Here's how the part is built. I have some questions about the finished solid (model axes, mm). A direction names the side the tool comes from. Round coordinates to 2 decimals unless told otherwise and drop trailing zeros. Loops run counter-clockwise (first coordinate to the right, second up) from the corner with the lowest first, then second, coordinate; pieces in that order, holes last. Notation, with made-up numbers: (83, 65.5) -> (115, 65.5) arc R21 cw to (115, 104.5) -> close; hole circle Ø6 at (41, 47.5). An arc over 180 degrees is marked (long way). One line per item, written item: value. Start each with the question number.
```python
from build123d import *

# Parameters (mm, degrees)
SKETCH1_W            = 40
SKETCH1_H            = 40
BOSS_EXTRUDE1_DEPTH  = 687
SKETCH1_4_W          = 40
SKETCH1_4_H          = 40
BOSS_EXTRUDE2_DEPTH  = 687
SKETCH1_5_W          = 40
SKETCH1_5_H          = 40
BOSS_EXTRUDE3_DEPTH  = 687
SKETCH1_6_W          = 40
SKETCH1_6_H          = 40
BOSS_EXTRUDE4_DEPTH  = 687
SKETCH1_7_W          = 820
SKETCH1_7_H          = 40
BOSS_EXTRUDE5_DEPTH  = 40
SKETCH1_8_W          = 40
SKETCH1_8_H          = 520
BOSS_EXTRUDE6_DEPTH  = 40
SKETCH1_9_W          = 820
SKETCH1_9_H          = 40
BOSS_EXTRUDE7_DEPTH  = 40
SKETCH1_10_W         = 40
SKETCH1_10_H         = 520
BOSS_EXTRUDE8_DEPTH  = 40
BOSS_EXTRUDE9_DEPTH  = 40
BOSS_EXTRUDE10_DEPTH = 40
BOSS_EXTRUDE11_DEPTH = 40
BOSS_EXTRUDE12_DEPTH = 40
SKETCH6_W            = 40
SKETCH6_H            = 40
BOSS_EXTRUDE13_DEPTH = 820
SKETCH7_W            = 40
SKETCH7_H            = 40
BOSS_EXTRUDE14_DEPTH = 520
SKETCH8_W            = 40
SKETCH8_H            = 40
BOSS_EXTRUDE15_DEPTH = 520
SKETCH9_R            = 12.5
BOSS_EXTRUDE16_DEPTH = 9


with BuildPart() as part:
    # Sketch1 → Boss-Extrude1 (new body)
    with BuildSketch(Plane.XY):
        with Locations((20, 580)):
            Rectangle(SKETCH1_W, SKETCH1_H)
    extrude(amount=BOSS_EXTRUDE1_DEPTH)



with BuildPart() as body_2:
    # Sketch1_4 → Boss-Extrude2 (new body)
    with BuildSketch(Plane.XY):
        with Locations((880, 580)):
            Rectangle(SKETCH1_4_W, SKETCH1_4_H)
    extrude(amount=BOSS_EXTRUDE2_DEPTH)


with BuildPart() as body_3:
    # Sketch1_5 → Boss-Extrude3 (new body)
    with BuildSketch(Plane.XY):
        with Locations((20, 20)):
            Rectangle(SKETCH1_5_W, SKETCH1_5_H)
    extrude(amount=BOSS_EXTRUDE3_DEPTH)


with BuildPart() as body_4:
    # Sketch1_6 → Boss-Extrude4 (new body)
    with BuildSketch(Plane.XY):
        with Locations((880, 20)):
            Rectangle(SKETCH1_6_W, SKETCH1_6_H)
    extrude(amount=BOSS_EXTRUDE4_DEPTH)


with BuildPart() as part_1:
    add(part.part)

    add(body_2.part)  # Boss-Extrude5 merges body 2
    # Sketch1_7 → Boss-Extrude5 (add)
    with BuildSketch(Plane.XY):
        with Locations((450, 580)):
            Rectangle(SKETCH1_7_W, SKETCH1_7_H)
    extrude(amount=BOSS_EXTRUDE5_DEPTH)


    add(body_3.part)  # Boss-Extrude6 merges body 3
    # Sketch1_8 → Boss-Extrude6 (add)
    with BuildSketch(Plane.XY):
        with Locations((20, 300)):
            Rectangle(SKETCH1_8_W, SKETCH1_8_H)
    extrude(amount=BOSS_EXTRUDE6_DEPTH)


    add(body_4.part)  # Boss-Extrude7 merges body 4
    # Sketch1_9 → Boss-Extrude7 (add)
    with BuildSketch(Plane.XY):
        with Locations((450, 20)):
            Rectangle(SKETCH1_9_W, SKETCH1_9_H)
    extrude(amount=BOSS_EXTRUDE7_DEPTH)

    # Sketch1_10 → Boss-Extrude8 (add)
    with BuildSketch(Plane.XY):
        with Locations((880, 300)):
            Rectangle(SKETCH1_10_W, SKETCH1_10_H)
    extrude(amount=BOSS_EXTRUDE8_DEPTH)

    # Sketch2 → Boss-Extrude9 (add)
    with BuildSketch(Plane(origin=(0, 600, 0), x_dir=(1, 0, 0), z_dir=(0, 1, 0))):
        Polygon((40, -140), (140, -40), (40, -40), align=None)
        Polygon((760, -40), (860, -140), (860, -40), align=None)
    extrude(amount=-BOSS_EXTRUDE9_DEPTH)

    # Sketch3 → Boss-Extrude10 (add)
    with BuildSketch(Plane.ZY):
        Polygon((40, 560), (40, 460), (140, 560), align=None)
        Polygon((40, 140), (40, 40), (140, 40), align=None)
    extrude(amount=-BOSS_EXTRUDE10_DEPTH)

    # Sketch4 → Boss-Extrude11 (add)
    with BuildSketch(Plane.XZ):
        Polygon((40, 140), (140, 40), (40, 40), align=None)
        Polygon((760, 40), (860, 140), (860, 40), align=None)
    extrude(amount=-BOSS_EXTRUDE11_DEPTH)

    # Sketch5 → Boss-Extrude12 (add)
    with BuildSketch(Plane(origin=(900, 0, 0), x_dir=(0, 0, -1), z_dir=(1, 0, 0))):
        Polygon((-140, 560), (-40, 460), (-40, 560), align=None)
        Polygon((-140, 40), (-40, 40), (-40, 140), align=None)
    extrude(amount=-BOSS_EXTRUDE12_DEPTH)

    # Sketch6 → Boss-Extrude13 (add)
    with BuildSketch(Plane.ZY.offset(-860)):
        with Locations((627, 580)):
            Rectangle(SKETCH6_W, SKETCH6_H)
    extrude(amount=BOSS_EXTRUDE13_DEPTH)

    # Sketch7 → Boss-Extrude14 (add)
    with BuildSketch(Plane.XZ.offset(-560)):
        with Locations((20, 627)):
            Rectangle(SKETCH7_W, SKETCH7_H)
    extrude(amount=BOSS_EXTRUDE14_DEPTH)

    # Sketch8 → Boss-Extrude15 (add)
    with BuildSketch(Plane.XZ.offset(-560)):
        with Locations((880, 627)):
            Rectangle(SKETCH8_W, SKETCH8_H)
    extrude(amount=BOSS_EXTRUDE15_DEPTH)

    # Sketch9 → Boss-Extrude16 (add)
    with BuildSketch(Plane(origin=(0, 0, 0), x_dir=(-1, 0, 0), z_dir=(0, 0, -1))):
        with Locations(Location((-880, 580, 0), (0, 0, 180))):
            Circle(SKETCH9_R)
        with Locations(Location((-880, 20, 0), (0, 0, 180))):
            Circle(SKETCH9_R)
        with Locations(Location((-20, 580, 0), (0, 0, 180))):
            Circle(SKETCH9_R)
        with Locations(Location((-20, 20, 0), (0, 0, 180))):
            Circle(SKETCH9_R)
    extrude(amount=BOSS_EXTRUDE16_DEPTH)


solid = part_1.part
```
Q1. I want a section at B-B on x = 116. Please give me the cut outline in (y, z), plus the area to 3 significant figures.
Q2. Will these pins go through, and if not, where does the flat tip stop? P1, Ø12, axis at x = 414, y = 577, coming from the -Z side; P2, Ø12, axis at x = 21.5, z = 669, coming from the -Y side; P3, Ø20, axis at x = 871.5, y = 305.5, coming from the +Z side.
Q3. I want a section at A-A on y = 83. Please give me the cut outline in (x, z), plus the area to 3 significant figures.
Q4. If I drill on line 1 along Z through (x, y) = (332, 575); line 2 along X through (y, z) = (35, 232); line 3 along Y through (x, z) = (857.5, 109), over which ranges is the centre line in solid material (lowest first)?
Q5. If we mould it in two halves opening along X, with no side actions, what happens to faces 1 (the flat face through (89, 20, 91)), 2 (the flat face through (20, 509, 89))? For each: released by +X, released by -X, zero draft, split by the parting line, or undercut.
Q6. I want a section at D-D on y = 580. Please give me the cut outline in (x, z), plus the area to 3 significant figures.
Q7. Which directions (+Z, -Z, +X, -X, +Y, -Y) give clear straight access to the entire face, cutting with the end or side of a thin tool? Please do faces 3 (the flat face through (446, 580, 40)), 4 (the flat face through (880, 511, 91)), 5 (the flat face through (809, 20, 89)), 6 (the flat face through (448, 35, 0)).
Q8. I want a section at C-C on z = 469. Please give me the cut outline in (x, y), plus the area to 3 significant figures.
Answers below:
1. outline: (0, 0) -> (40, 0) -> (40, 64) -> (0, 64) -> close; (560, 0) -> (600, 0) -> (600, 64) -> (560, 64) -> close; (560, 607) -> (600, 607) -> (600, 647) -> (560, 647) -> close
1. area: 6,720 mm^2
2. P1: stops at z = 0
2. P2: stops at y = 0
2. P3: stops at z = 647
3. outline: (0, 0) -> (40, 0) -> (40, 97) -> (0, 97) -> close; (0, 607) -> (40, 607) -> (40, 647) -> (0, 647) -> close; (860, 0) -> (900, 0) -> (900, 97) -> (860, 97) -> close; (860, 607) -> (900, 607) -> (900, 647) -> (860, 647) -> close
3. area: 11,000 mm^2
4. line 1: z = 0 to 40, 607 to 647
4. line 2: x = 0 to 40, 860 to 900
4. line 3: y = 0 to 40, 560 to 600
5. face 1: undercut
5. face 2: zero draft
6. outline: (0, 0) -> (7.5, 0) -> (7.5, -9) -> (32.5, -9) -> (32.5, 0) -> (867.5, 0) -> (867.5, -9) -> (892.5, -9) -> (892.5, 0) -> (900, 0) -> (900, 687) -> (860, 687) -> (860, 647) -> (40, 647) -> (40, 687) -> (0, 687) -> close; hole (40, 140) -> (140, 40) -> (760, 40) -> (860, 140) -> (860, 607) -> (40, 607) -> close
6. area: 131,000 mm^2
7. face 3: +Y, -Y
7. face 4: +X, -X
7. face 5: +Z, +Y, -Y
7. face 6: -Z
8. outline: (0, 0) -> (40, 0) -> (40, 40) -> (0, 40) -> close; (0, 560) -> (40, 560) -> (40, 600) -> (0, 600) -> close; (860, 0) -> (900, 0) -> (900, 40) -> (860, 40) -> close; (860, 560) -> (900, 560) -> (900, 600) -> (860, 600) -> close
8. area: 6,400 mm^2
